```python
from build123d import *

# Parameters (mm, degrees)
SKETCH1_W           = 32
SKETCH1_H           = 32
SKETCH1_R           = 1.3
SKETCH1_R_2         = 1.4
SKETCH1_R_3         = 3.5
BOSS_EXTRUDE1_DEPTH = 8
SKETCH2_R           = 12
CUT_EXTRUDE1_DEPTH  = 2.5
FILLET1_R           = 2
SKETCH3_R           = 3
CUT_EXTRUDE2_DEPTH  = 3


with BuildPart() as part:
    # Sketch1 → Boss-Extrude1 (new body)
    with BuildSketch(Plane(origin=(0, 0, 0), x_dir=(1, 0, 0), z_dir=(0, 1, 0))):
        with Locations((16, 16)):
            Rectangle(SKETCH1_W, SKETCH1_H)
        with Locations((3.5, 16)):
            Circle(SKETCH1_R, mode=Mode.SUBTRACT)
        with Locations((4.5, 27.5)):
            Circle(SKETCH1_R_2, mode=Mode.SUBTRACT)
        with Locations((27.5, 27.5)):
            Circle(SKETCH1_R_2, mode=Mode.SUBTRACT)
        with Locations((27.5, 4.5)):
            Circle(SKETCH1_R_2, mode=Mode.SUBTRACT)
        with Locations((4.5, 4.5)):
            Circle(SKETCH1_R_2, mode=Mode.SUBTRACT)
        with Locations((28.5, 16)):
            Circle(SKETCH1_R, mode=Mode.SUBTRACT)
        with Locations((16, 16)):
            Circle(SKETCH1_R_3, mode=Mode.SUBTRACT)
    extrude(amount=BOSS_EXTRUDE1_DEPTH)

    # Sketch2 → Cut-Extrude1 (cut)
    with BuildSketch(Plane(origin=(0, 8, 0), x_dir=(1, 0, 0), z_dir=(0, 1, 0))):
        with Locations((16, 16)):
            Circle(SKETCH2_R)
    extrude(amount=-CUT_EXTRUDE1_DEPTH, mode=Mode.SUBTRACT)

    # Fillet1
    fillet1_edges = [part.edges().sort_by_distance(p)[0] for p in [
        (0, 4, -32),
        (32, 4, -32),
        (32, 4, 0),
        (0, 4, 0),
    ]]
    fillet(fillet1_edges, radius=FILLET1_R)

    # Sketch3 → Cut-Extrude2 (cut)
    with BuildSketch(Plane.XZ):
        with Locations((27.5, -4.5)):
            Circle(SKETCH3_R)
        with Locations((27.5, -27.5)):
            Circle(SKETCH3_R)
        with Locations((4.5, -27.5)):
            Circle(SKETCH3_R)
        with Locations((4.5, -4.5)):
            Circle(SKETCH3_R)
    extrude(amount=-CUT_EXTRUDE2_DEPTH, mode=Mode.SUBTRACT)


solid = part.part
```
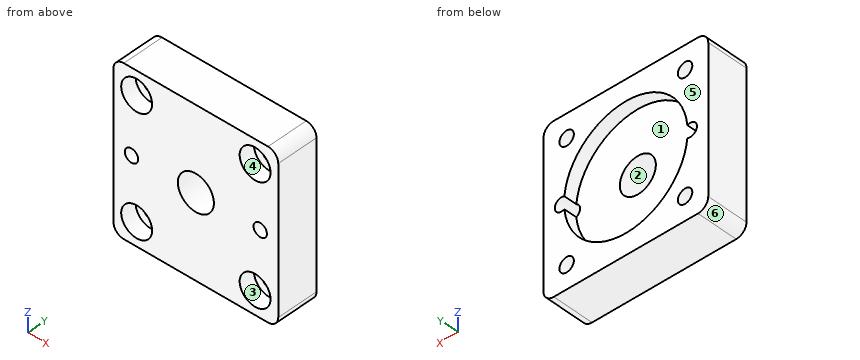
Design review of the part built by this model. Coordinates are the model's own, in mm. Face numbers are marked on the shaded views. A direction names the side the tool comes from. Coordinates: 2 decimals unless noted, no trailing zeros. Loops run counter-clockwise (first coordinate to the right, second up) from the corner with the lowest first, then second, coordinate; pieces in that order, holes last.
Q1. We need section A-A on x = 16. State the section outline as (y, z) points.
Reported:
outline: (0, -32) - (8, -32) - (8, -28) - (5.5, -28) - (5.5, -19.5) - (0, -19.5) - close; (0, -12.5) - (5.5, -12.5) - (5.5, -4) - (8, -4) - (8, 0) - (0, 0) - close
Q2. For pin 1 (8 mm diameter, centred on x = 16, z = -16, fed in from +Y); pin 2 (2.5 mm diameter, centred on x = 4.5, z = -27.5, fed in from -Y); pin 3 (1.8 mm diameter, centred on x = 3.5, z = -4.5, fed in from -Y), all flat-tipped, find the tip position at first contact; note any pin that passes through.
Reported:
pin 1: stops at y = 5.5
pin 2: passes through
pin 3: stops at y = 3
Q3. We need section C-C on z = -16. State the section outline as (x, y) points.
Reported:
outline: (0, 0) - (2.2, 0) - (2.2, 8) - (0, 8) - close; (4.8, 0) - (12.5, 0) - (12.5, 5.5) - (4.8, 5.5) - close; (19.5, 0) - (27.2, 0) - (27.2, 5.5) - (19.5, 5.5) - close; (29.8, 0) - (32, 0) - (32, 8) - (29.8, 8) - close
Q4. We need section B-B on y = 7. State the section outline as (x, z) points, and give its area (3 significant figures).
Reported:
outline: (0, -30) arc R2 ccw to (2, -32) - (30, -32) arc R2 ccw to (32, -30) - (32, -2) arc R2 ccw to (30, 0) - (2, 0) arc R2 ccw to (0, -2) - close; hole circle Ø2.8 at (4.5, -27.5); hole circle Ø2.8 at (4.5, -4.5); hole (4.06, -17.17) arc R12 ccw to (27.94, -17.17) arc R1.3 ccw (long way) to (27.94, -14.83) arc R12 ccw to (4.06, -14.83) arc R1.3 ccw (long way) to start; hole circle Ø2.8 at (27.5, -27.5); hole circle Ø2.8 at (27.5, -4.5)
area: 536 mm2
Q5. The part is to be moulded in two halves that separate along X. For the marked faces 4, 5 and 6, say which applies: +X half, -X half, draft (parallel to the pull), parting line (faces both ways), or undercut.
Reported:
face 4: undercut
face 5: draft
face 6: -X half
Q6. Tool access review of the marked faces 1, 2 and 3: name each direction out of +Z, -Z, +X, -X, +Y, -Y from which nothing blocks a thin tool from reaching the whole face with its end or side.
Reported:
face 1: +Y
face 2: +Y, -Y
face 3: -Y
Q7. We need section D-D on z = -5.5. State the section outline as (x, y) points.
Reported:
outline: (0, 0) - (1.67, 0) - (1.67, 3) - (3.52, 3) - (3.52, 8) - (0, 8) - close; (5.48, 3) - (7.33, 3) - (7.33, 0) - (24.67, 0) - (24.67, 3) - (26.52, 3) - (26.52, 8) - (21.81, 8) - (21.81, 5.5) - (10.19, 5.5) - (10.19, 8) - (5.48, 8) - close; (28.48, 3) - (30.33, 3) - (30.33, 0) - (32, 0) - (32, 8) - (28.48, 8) - close
Q8. To check wall thickness, follow line 1 (X direction, y = 5.3, z = -27.5); line 2 (Z direction, x = 16, y = 4); line 3 (Z direction, x = 28.5, y = 4). State the ranges of each line that lie inside material, in increasing order.
Reported:
line 1: x = 0 to 3.1, 5.9 to 26.1, 28.9 to 32
line 2: z = -32 to -19.5, -12.5 to 0
line 3: z = -32 to -28.48, -26.52 to -17.3, -14.7 to -5.48, -3.52 to 0
